CAD build for the part. Positions are in the model's coordinates, mm. A direction names the side the tool comes from. Give positions to 0.01 mm unless a question says otherwise; leave off trailing zeros. Loops run counter-clockwise (first coordinate to the right, second up) from the corner with the lowest first, then second, coordinate; pieces in that order, holes last.
Item 1: Saw through at A-A on x = -61. Give the cut face in (y, z), plus the area to 3 significant figures.
Item 2: Saw through at B-B on z = -3.75. Give the number of separate pieces and of enclosed holes in the cut face, plus the area to 3 significant figures.
Item 3: Which spindle directions (+Z, -Z, +X, -X, +Y, -Y) get a long thin tool onto all of the face, cutting with end or side? Do faces 1 (the flat face through (60, 6, -3)), 2 (the flat face through (-25, 59, -3)), 3 (the flat face through (19.9, 60, -5)), 4 (the flat face through (3.05, 23, -3)), 5 (the flat face through (-1, 11, 0)). Say none if no direction does.
Item 4: Mould opens along X. For faces 6 (the flat face through (91, 62, -3)), 7 (the flat face through (89.03, 40.74, -3.45)), 8 (the flat face through (-3.05, 23, -3)), 9 (the cylindrical face through (-96.416, 60.496, -3.549)) say: released by +X, released by -X, zero draft, split by the parting line, or undercut.
Item 5: Drop flat-ended pins along their axis: P1, Ø1.5, axis at x = -37.5, z = -1.5, coming from the +Y side; P2, Ø5, axis at x = -65.14, y = 12.57, coming from the -Z side; P3, Ø1, axis at y = 0.5, z = -3.5, coming from the +X side; P4, Ø3, axis at x = -21.5, z = -3.5, coming from the +Y side. Give the stop position or say it passes through.
Item 6: Probe probe 1 along Y at (x, z) = (-41, -3.5); probe 2 along X at (y, z) = (39, -1); probe 3 along X at (y, z) = (78, -4.5). List the from-to ranges inside material, lowest first.
from build123d import *

# Parameters (mm, degrees)
F0_R     = 1.6
F0_R_2   = 4.1
F0_R_3   = 1.75
F1_DEPTH = 7
F2_R     = 5
F5_R     = 8
F0_W     = 19.9004877359
F0_H     = 28.2499268651
F6_DEPTH = 2.5


# Not quite as in the source:
# - two fillets or chamfers of one size are made in one step
# - a feature names something its author has since deleted; it is built from what else it names


with BuildPart() as f1:
    # F0 (on Top) → F1 (new body)
    with BuildSketch(Plane.XY):
        with BuildLine():
            Line((-80, 31.2532794885), (-80, 6))
            Line((-80, 6), (-39.382737335, 6))
            ThreePointArc((-39.382737335, 6), (-35.7696607995, -18.9033897988), (-18, -36.721142199))
            Line((-18, -36.721142199), (-18, -63))
            Line((-18, -63), (0, -63))
            Line((0, -63), (0, -56.6))
            ThreePointArc((0, -56.6), (-1.6, -55), (0, -53.4))
            Line((0, -53.4), (0, -23.1440107676))
            ThreePointArc((0, -23.1440107676), (-2.1566756826, -22.2506864502), (-3.05, -20.0940107676))
            Line((-3.05, -20.0940107676), (-3.05, -14.0940107676))
            ThreePointArc((-3.05, -14.0940107676), (-2.1566756826, -11.937335085), (0, -11.0440107676))
            Line((0, -11.0440107676), (0, 17.0440107676))
            ThreePointArc((0, 17.0440107676), (-2.1566756826, 17.937335085), (-3.05, 20.0940107676))
            Line((-3.05, 20.0940107676), (-3.05, 26.0940107676))
            ThreePointArc((-3.05, 26.0940107676), (-2.1566756826, 28.2506864502), (0, 29.1440107676))
            Line((0, 29.1440107676), (0, 38))
            Line((0, 38), (0, 46.1897078156))
            Line((0, 46.1897078156), (-19.9004877359, 46.1897078156))
            Line((-19.9004877359, 46.1897078156), (-19.9004877359, 74.4396346807))
            Line((-19.9004877359, 74.4396346807), (0, 74.4396346807))
            Line((0, 74.4396346807), (0, 83))
            Line((0, 83), (-25, 83))
            Line((-25, 83), (-25, 38))
            Line((-25, 38), (-73.253, 38))
            Line((-73.253, 38), (-84.158, 50))
            Line((-84.158, 50), (-84.158, 62))
            Line((-84.158, 62), (-97.842, 62))
            Line((-97.842, 62), (-97.842, 50))
            Line((-97.842, 50), (-80, 31.2532794885))
        make_face()
        with Locations((-10.5, -55)):
            Circle(F0_R, mode=Mode.SUBTRACT)
        with BuildLine():
            ThreePointArc((-21.0730762114, -15.6883828653), (-25.2394536929, -14.5720053838), (-24.1230762114, -10.4056279022))
            Line((-24.1230762114, -10.4056279022), (-18.9269237886, -7.4056279022))
            ThreePointArc((-18.9269237886, -7.4056279022), (-14.7605463071, -8.5220053838), (-15.8769237886, -12.6883828653))
            Line((-15.8769237886, -12.6883828653), (-21.0730762114, -15.6883828653))
        make_face(mode=Mode.SUBTRACT)
        with Locations((-73.6379495263, 12.566276442)):
            Circle(F0_R, mode=Mode.SUBTRACT)
        with Locations((-73.6379495263, 18.566276442)):
            Circle(F0_R, mode=Mode.SUBTRACT)
        with Locations((-73.6379495263, 25.566276442)):
            Circle(F0_R, mode=Mode.SUBTRACT)
        with Locations((-73.6379495263, 31.566276442)):
            Circle(F0_R, mode=Mode.SUBTRACT)
        with Locations((-65.1379495263, 12.566276442)):
            Circle(F0_R, mode=Mode.SUBTRACT)
        with Locations((-65.1379495263, 18.566276442)):
            Circle(F0_R, mode=Mode.SUBTRACT)
        with Locations((-56.6379495263, 12.566276442)):
            Circle(F0_R, mode=Mode.SUBTRACT)
        with Locations((-56.6379495263, 18.566276442)):
            Circle(F0_R, mode=Mode.SUBTRACT)
        with Locations((-65.1379495263, 25.566276442)):
            Circle(F0_R, mode=Mode.SUBTRACT)
        with Locations((-56.6379495263, 25.566276442)):
            Circle(F0_R, mode=Mode.SUBTRACT)
        with Locations((-48.1379495263, 12.566276442)):
            Circle(F0_R, mode=Mode.SUBTRACT)
        with Locations((-48.1379495263, 18.566276442)):
            Circle(F0_R, mode=Mode.SUBTRACT)
        with Locations((-39.6379495263, 12.566276442)):
            Circle(F0_R, mode=Mode.SUBTRACT)
        with Locations((-39.6379495263, 18.566276442)):
            Circle(F0_R, mode=Mode.SUBTRACT)
        with Locations((-48.1379495263, 25.566276442)):
            Circle(F0_R, mode=Mode.SUBTRACT)
        with Locations((-39.6379495263, 25.566276442)):
            Circle(F0_R, mode=Mode.SUBTRACT)
        with Locations((-65.1379495263, 31.566276442)):
            Circle(F0_R, mode=Mode.SUBTRACT)
        with Locations((-56.6379495263, 31.566276442)):
            Circle(F0_R, mode=Mode.SUBTRACT)
        with Locations((-48.1379495263, 31.566276442)):
            Circle(F0_R, mode=Mode.SUBTRACT)
        with Locations((-39.6379495263, 31.566276442)):
            Circle(F0_R, mode=Mode.SUBTRACT)
        with Locations((-91, 56)):
            Circle(F0_R_2, mode=Mode.SUBTRACT)
        with BuildLine():
            Line((-18.9269237886, 13.4056279022), (-24.1230762114, 16.4056279022))
            ThreePointArc((-24.1230762114, 16.4056279022), (-25.2394536929, 20.5720053838), (-21.0730762114, 21.6883828653))
            Line((-21.0730762114, 21.6883828653), (-15.8769237886, 18.6883828653))
            ThreePointArc((-15.8769237886, 18.6883828653), (-14.7605463071, 14.5220053838), (-18.9269237886, 13.4056279022))
        make_face(mode=Mode.SUBTRACT)
        with Locations((-20, 43)):
            Circle(F0_R_3, mode=Mode.SUBTRACT)
        with Locations((-20, 78)):
            Circle(F0_R_3, mode=Mode.SUBTRACT)
    extrude(amount=-F1_DEPTH)

    # F2
    f2_edges = [f1.edges().sort_by_distance(p)[0] for p in [
        (-39.382737, 6, -3.5),
        (-80, 6, -3.5),
        (-18, -36.721142, -3.5),
        (-18, -63, -3.5),
        (-73.253, 38, -3.5),
        (-84.158, 50, -3.5),
        (-84.158, 62, -3.5),
        (-97.842, 62, -3.5),
        (-97.842, 50, -3.5),
        (-80, 31.253279, -3.5),
        (-25, 38, -3.5),
    ]]
    fillet(f2_edges, radius=F2_R)

    # F3: F1 across plane


with BuildPart() as f1_1:
    add(f1.part)
    add(f1.part.mirror(Plane.YZ))

    # F5
    f5_edges = [f1_1.edges().sort_by_distance(p)[0] for p in [
        (-25, 83, -3.5),
        (25, 83, -3.5),
    ]]
    fillet(f5_edges, radius=F5_R)

    # F0 (on Top) → F6 (join)
    with BuildSketch(Plane.XY):
        with Locations((9.9502438679, 60.3146712482)):
            Rectangle(F0_W, F0_H)
        with Locations((-9.9502438679, 60.3146712482)):
            Rectangle(F0_W, F0_H)
    extrude(amount=-F6_DEPTH)


solid = f1_1.part
Results below:
1. outline: (6, -7) - (38, -7) - (38, 0) - (6, 0) - close
1. area: 224 mm2
2. separate pieces: 1
2. enclosed holes: 56
2. area: 9,930 mm2
3. face 1: +Z, -Z, +X, -Y
3. face 2: +Z, -Z, +Y
3. face 3: -Z
3. face 4: +Z, -Z
3. face 5: +Z, +X, -X, +Y, -Y
4. face 6: zero draft
4. face 7: released by +X
4. face 8: undercut
4. face 9: released by -X
5. P1: stops at y = 38
5. P2: stops at z = -7
5. P3: stops at x = 39.99
5. P4: stops at y = 82.42
6. probe 1: y = 4.06 to 11.73, 13.41 to 17.73, 19.41 to 24.73, 26.41 to 30.73, 32.41 to 38
6. probe 2: x = -87.37 to -74.04, -27 to 27, 74.04 to 87.37
6. probe 3: x = -24.42 to -21.75, -18.25 to 18.25, 21.75 to 24.42
